Could you check a few things on this drawing? It's one solid part, dimensions in mm from its lowest x, y, z. Give positions to 0.01 mm unless a question says otherwise; leave off trailing zeros. Loops run counter-clockwise (first coordinate to the right, second up) from the corner with the lowest first, then second, coordinate; pieces in that order, holes last. Notation, with made-up numbers: (81, -9) -> (102, -9) arc R24 ccw to (102, 13) -> close; hole circle Ø4 at (-17.75, 11.25). An arc over 180 degrees is marked (long way). Use CSV: the item, a comma, the result in double quotes.
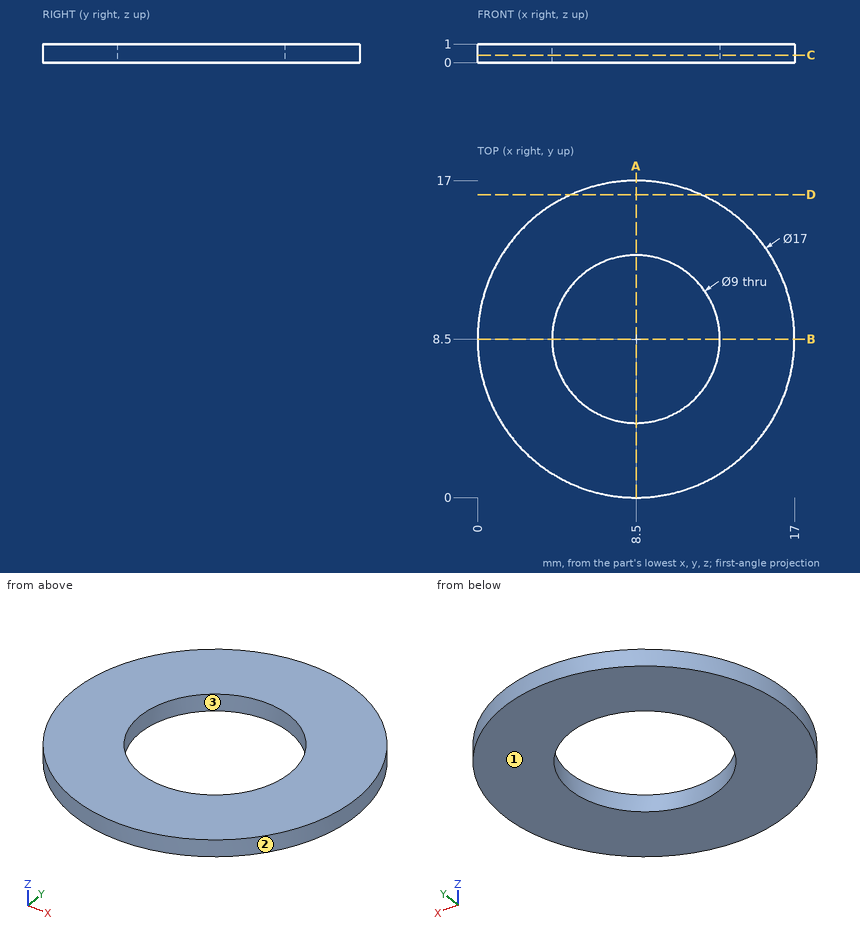
(1) If we section it at D-D, the plane y = 16.25: Write out the boundary of the cut face in (x, z), then the cut area to 3 significant figures.
Answer sheet:
outline,"(5.01, 0) -> (11.99, 0) -> (11.99, 1) -> (5.01, 1) -> close"
area,"6.98 mm2"
(2) If I drill on L1, parallel to X at y = 8.5, z = 0.2; L2, parallel to Y at x = 10, z = 0.6, over which ranges is the centre line in solid material (lowest first)? Write a range as from..to.
Answer sheet:
L1,"x = 0..4, 13..17"
L2,"y = 0.13..4.26, 12.74..16.87"
(3) If we section it at A-A, the plane x = 8.5: Write out the boundary of the cut face in (y, z).
Answer sheet:
outline,"(0, 0) -> (4, 0) -> (4, 1) -> (0, 1) -> close; (13, 0) -> (17, 0) -> (17, 1) -> (13, 1) -> close"
(4) If we section it at C-C, the plane z = 0.4: Write out the boundary of the cut face in (x, y), then the cut area to 3 significant figures.
Answer sheet:
outline,"circle Ø17 at (8.5, 8.5); hole circle Ø9 at (8.5, 8.5)"
area,"163 mm2"
(5) We'd pull the mould along X, two halves only. Please class the marked faces 1, 2 and 3: released by +X, released by -X, zero draft, split by the parting line, or undercut.
Answer sheet:
face 1,"zero draft"
face 2,"split by the parting line"
face 3,"undercut"
